Can you work these out from the model? Positions are in its coordinate system, mm. A direction names the side the tool comes from. Give positions to 0.01 mm unless a question says otherwise; leave off trailing zeros. Order: outer loops, then holes, each group sorted by start corner. A loop starts at its lowest first (then second) coordinate and runs counter-clockwise, first axis right, second up. Notation, with made-up numbers: (5, -12.75) - (44, -12.75) arc R21 ccw to (44, -3.75) - close; hole circle Ø9 at (81, -28). An arc over 180 degrees is marked (long way). Return JSON: item names as keys, results as strings.
```python
from build123d import *

# Parameters (mm, degrees)
SKETCH1_R               = 2.54
BOSS_EXTRUDE1_DEPTH     = 38.1
CUT_EXTRUDE1_DEPTH      = 3.81
CUT_EXTRUDE1_DEPTH_BACK = 3.81
SKETCH4_R               = 5.08


with BuildPart() as part:
    # Sketch1 → Boss-Extrude1 (new body)
    with BuildSketch(Plane(origin=(0, 0, 0), x_dir=(0, 0, -1), z_dir=(1, 0, 0))):
        with BuildLine():
            Line((11.199311053, -5.988775495), (0.344819113, -26.287220755))
            ThreePointArc((0.344819113, -26.287220755), (-0.103387784, -26.766158861), (-0.730789632, -26.957569556))
            Line((-0.730789632, -26.957569556), (-94.938797587, -30.247385686))
            ThreePointArc((-94.938797587, -30.247385686), (-96.22161935, -29.25926293), (-95.4910689, -27.814162831))
            Line((-95.4910689, -27.814162831), (-5.079489514, 11.639965046))
            ThreePointArc((-5.079489514, 11.639965046), (-2.594459858, 12.432167069), (0, 12.7))
            Line((0, 12.7), (11.43, 12.7))
            ThreePointArc((11.43, 12.7), (12.328025612, 12.328025612), (12.7, 11.43))
            Line((12.7, 11.43), (12.7, 0))
            ThreePointArc((12.7, 0), (12.31911625, -3.086968547), (11.199311053, -5.988775495))
        make_face()
        with Locations(Location((0, 0, 0), (0, 0, 180))):
            Circle(SKETCH1_R, mode=Mode.SUBTRACT)
    extrude(amount=BOSS_EXTRUDE1_DEPTH)

    # Sketch4 → Cut-Extrude1 (cut, two sides: drawn at the far end of the back side and taken through both)
    with BuildSketch(Plane(origin=(19.05, 0, 0), x_dir=(0, 0, -1), z_dir=(1, 0, 0)).offset(-CUT_EXTRUDE1_DEPTH_BACK)):
        with BuildLine():
            Line((-5.08, 25.792214679), (-5.08, 0))
            ThreePointArc((-5.08, 0), (0, 5.08), (5.08, 0))
            ThreePointArc((5.08, 0), (1.314800749, -4.906903198), (-4.399409051, -2.54))
            Line((-4.399409051, -2.54), (14.172067989, -34.706741806))
            Line((14.172067989, -34.706741806), (14.172067989, 25.792214679))
            Line((14.172067989, 25.792214679), (-5.08, 25.792214679))
        make_face()
        Circle(SKETCH4_R)
    extrude(amount=CUT_EXTRUDE1_DEPTH + CUT_EXTRUDE1_DEPTH_BACK, mode=Mode.SUBTRACT)


solid = part.part
```
1. Suppose I cut it at A-A (x = 34.5). List the corners of the cut face in (y, z) for me, plus the area to 3 significant figures.
Checks:
{"outline": "(-30.25, 94.94) - (-26.96, 0.73) arc R1.27 ccw to (-26.29, -0.34) - (-5.99, -11.2) arc R12.7 ccw to (0, -12.7) - (11.43, -12.7) arc R1.27 ccw to (12.7, -11.43) - (12.7, 0) arc R12.7 ccw to (11.64, 5.08) - (-27.81, 95.49) arc R1.27 ccw to start; hole circle Ø5.08 at (0, 0)", "area": "2,390 mm^2"}
2. Suppose I cut it at C-C (y = -11.5). List the corners of the cut face in (x, z) for me, plus the area to 3 significant figures.
Checks:
{"outline": "(0, -8.25) - (15.24, -8.25) - (15.24, -0.77) - (22.86, -0.77) - (22.86, -8.25) - (38.1, -8.25) - (38.1, 58.11) - (0, 58.11) - close", "area": "2,470 mm^2"}
3. On a 3-axis mill with a long thin cutter (end or side, diameter ignored), from which of +Z, -Z, +X, -X, +Y, -Y can I reach the whole of each face in a straight line? I mean faces 5 (the face through (19, -1.3, 4.91)), 6 (the face through (23.017, -15.996, -5.848)). Say none if no direction works.
Checks:
{"face 5": "-Z, +Y", "face 6": "-Z, +X, -X, -Y"}
4. For pin 1 Ø12 at (x, z) = (21, 40) entering from +Y; pin 2 Ø3 at (x, y) = (14, -26) entering from -Z; pin 3 Ø8 at (x, y) = (12, -18.5) entering from +Z, each with a flat end and sliding along its axis, tell me the tip position at first contact or that it passes through.
Checks:
{"pin 1": "y = -0.98", "pin 2": "z = -1.3", "pin 3": "z = 83.31"}
5. Thinking about a two-plate mould opening in X: for faces 1 (the face through (0, -13, 29)), 2 (the face through (15.24, 1, -4)), 3 (the face through (30.37, -2.52, -0.33)), 4 (the face through (38.1, -13, 29)), which applies, +X half, -X half, draft (parallel to the pull), parting line (faces both ways), or undercut?
Checks:
{"face 1": "-X half", "face 2": "undercut", "face 3": "draft", "face 4": "+X half"}
6. If I drill on L1, parallel to Y at x = 12, z = 0; L2, parallel to Z at x = 8, y = -21; L3, parallel to Y at x = 21, z = 90.5, over which ranges is the centre line in solid material (lowest first)? Write a range as [from, to].
Checks:
{"L1": "[-26.69, -2.54], [2.54, 12.7]", "L2": "[-3.17, 79.88]", "L3": "[-30.09, -25.64]"}
7. Suppose I cut it at D-D (z = 14). List the corners of the cut face in (x, y) for me.
Checks:
{"outline": "(0, -27.42) - (38.1, -27.42) - (38.1, 7.75) - (0, 7.75) - close"}
8. Suppose I cut it at B-B (x = 21). List the corners of the cut face in (y, z) for me.
Checks:
{"outline": "(-30.25, 94.94) - (-26.96, 0.73) arc R1.27 ccw to (-26.29, -0.34) - (-18.22, -4.66) - (-2.54, 4.4) arc R5.08 cw to (0, 5.08) - (11.64, 5.08) - (-27.81, 95.49) arc R1.27 ccw to start"}
